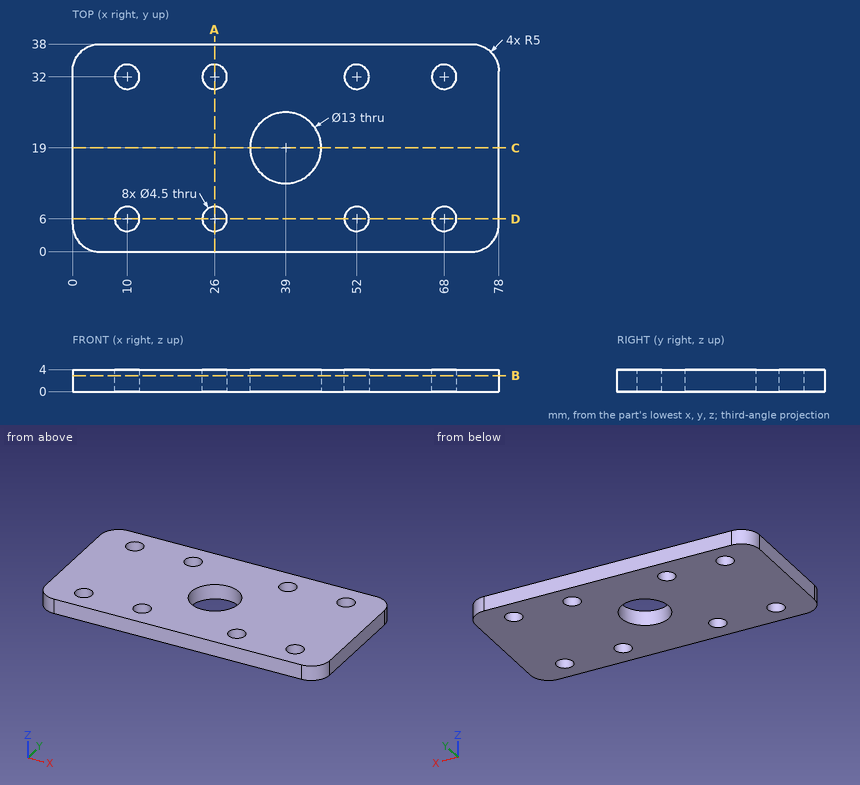
Geometry check sheet. Reference: drawing and pictorial views, mm from the part's lowest x, y, z. Give positions to 0.01 mm unless a question says otherwise; leave off trailing zeros. Order: outer loops, then holes, each group sorted by start corner. A loop starts at its lowest first (then second) coordinate and runs counter-clockwise, first axis right, second up. Notation, with made-up numbers: (-30, -5) - (-22, -5) arc R13 cw to (-22, 18) - close; hole circle Ø2 at (-31, -28). An arc over 180 degrees is marked (long way). Use one line per item in the form item = value.
1) Sectioned sample at B-B (z = 2.9). Count the separate pieces of the cut face and the enclosed holes in it, and give its area (3 significant figures).
Working result:
separate_pieces = 1
enclosed_holes = 9
area = 2,680 mm^2
2) Sectioned sample at D-D (y = 6). Record the boundary of the cut face in (x, z), and give its area (3 significant figures).
Working result:
outline = (0, 0) - (7.75, 0) - (7.75, 4) - (0, 4) - close; (12.25, 0) - (23.75, 0) - (23.75, 4) - (12.25, 4) - close; (28.25, 0) - (49.75, 0) - (49.75, 4) - (28.25, 4) - close; (54.25, 0) - (65.75, 0) - (65.75, 4) - (54.25, 4) - close; (70.25, 0) - (78, 0) - (78, 4) - (70.25, 4) - close
area = 240 mm^2
3) Material ranges on probe 1 along Y at (x, z) = (10, 1.25); probe 2 along X at (y, z) = (31.5, 1); probe 3 along X at (y, z) = (7.5, 1.15), recorded low to high. Write a range as from..to.
Working result:
probe_1 = 0..3.75, 8.25..29.75, 34.25..38
probe_2 = 0..7.81, 12.19..23.81, 28.19..49.81, 54.19..65.81, 70.19..78
probe_3 = 0..8.32, 11.68..24.32, 27.68..50.32, 53.68..66.32, 69.68..78
4) Sectioned sample at A-A (x = 26). Record the boundary of the cut face in (y, z), and give its area (3 significant figures).
Working result:
outline = (0, 0) - (3.75, 0) - (3.75, 4) - (0, 4) - close; (8.25, 0) - (29.75, 0) - (29.75, 4) - (8.25, 4) - close; (34.25, 0) - (38, 0) - (38, 4) - (34.25, 4) - close
area = 116 mm^2
5) Depth check by flat-ended pin: pin 1 Ø7 at (x, y) = (52, 32) entering from +Z. Enter the tip coordinate at first touch or a pass-through.
Working result:
pin_1 = 4
6) Sectioned sample at C-C (y = 19). Record the boundary of the cut face in (x, z).
Working result:
outline = (0, 0) - (32.5, 0) - (32.5, 4) - (0, 4) - close; (45.5, 0) - (78, 0) - (78, 4) - (45.5, 4) - close
